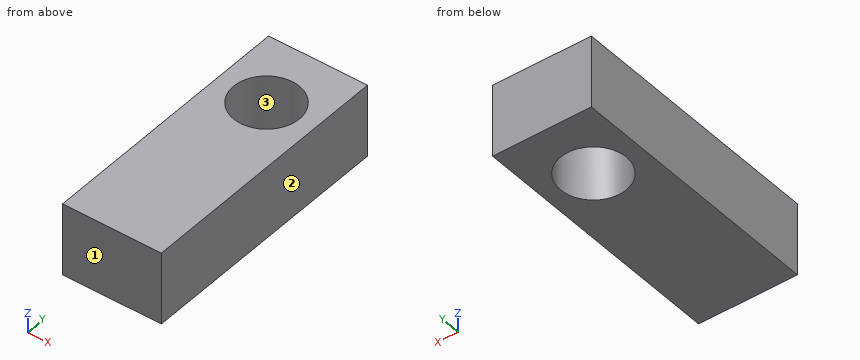
Autodesk Inventor part; units mm, degrees
ref_plane "YZ Plane" through (0, 0, 0) normal (1, 0, 0) x (0, 1, 0)
ref_plane "XZ Plane" through (0, 0, 0) normal (0, 1, 0) x (-1, 0, 0)
ref_plane "XY Plane" through (0, 0, 0) normal (0, 0, 1) x (1, 0, 0)
sketch "Sketch1" plane through (0, 0, 0) normal (0, 0, 1) x (1, 0, 0)
  line L0 (-7.5, 40) -> (7.5, 40)
  line L1 (7.5, 40) -> (7.5, 0)
  line L2 (7.5, 0) -> (-7.5, 0)
  line L3 (-7.5, 0) -> (-7.5, 40)
  line L4 (-10.7602, 0) -> (12.0613, 0)
  line L5 (0, -8) -> (0, 48)
  point P0 (0, 0)
  dimension "d4" = 7.5
  dimension "d5" = 7.5
  dimension "d6" = 40
  dimension "d7" = 0
extrude "Extrusion1" add sketch "Sketch1" along normal blind 11
sketch "Sketch3" plane through (-7.5, 0, 0) normal (0, -1, 0) x (1, 0, 0)
  line L0 (0, 0) -> (0, 11)
  line L1 (0, 5.5) -> (13.8011, 5.5)
  line L2 (0, 11) -> (15, 11)
  circle A0 centre (5, 5.5) radius 1
  point P0 (7.5, 0)
  dimension "d11" = 5.5
  dimension "d12" = 2
sketch "Sketch4" plane through (0, 0, 11) normal (0, 0, 1) x (1, 0, 0)
  circle A0 centre (0, 30) radius 5
  line L0 (-7.5, 0) -> (7.5, 0)
  point P0 (0, 0)
  dimension "d13" = 10
  dimension "d14" = 30
extrude "Extrusion3" cut sketch "Sketch4" against normal through all
properties part number "mallet_support"
The model under review builds one solid part; all positions refer to its coordinate system, in mm. Face numbers are marked on the shaded views. Round coordinates to 2 decimals unless told otherwise and drop trailing zeros. Loops run counter-clockwise (first coordinate to the right, second up) from the corner with the lowest first, then second, coordinate; pieces in that order, holes last. Notation, with made-up numbers: (43, 1) -> (94, 1) arc R21 cw to (94, 17) -> close; hole circle Ø1 at (-4, -24). An arc over 180 degrees is marked (long way). Answer as CSV lines item,"result".
1) To check wall thickness, follow line 1 along Y through (x, z) = (0.25, 5.5); line 2 along Y through (x, z) = (-3.5, 1.25); line 3 along X through (y, z) = (29.5, 7.25). State the ranges of each line that lie inside material, in increasing order. Write a range as from..to.
Geometry results:
line 1,"y = 0..25.01, 34.99..40"
line 2,"y = 0..26.43, 33.57..40"
line 3,"x = -7.5..-4.97, 4.97..7.5"
2) Add section A-A on z = 1.5. Write out the cut boundary in (x, y).
Geometry results:
outline,"(-7.5, 0) -> (7.5, 0) -> (7.5, 40) -> (-7.5, 40) -> close; hole circle Ø10 at (0, 30)"
3) Add section B-B on y = 30. Write out the cut boundary in (x, z).
Geometry results:
outline,"(-7.5, 0) -> (-5, 0) -> (-5, 11) -> (-7.5, 11) -> close; (5, 0) -> (7.5, 0) -> (7.5, 11) -> (5, 11) -> close"
4) Add section C-C on x = 0. Write out the cut boundary in (y, z).
Geometry results:
outline,"(0, 0) -> (25, 0) -> (25, 11) -> (0, 11) -> close; (35, 0) -> (40, 0) -> (40, 11) -> (35, 11) -> close"
5) Draft analysis for pull direction Y (two halves, no side actions). For the marked faces 1, 2 and 3, state which applies: pulls with the +Y half, pulls with the -Y half, needs draft (parallel to the pull), parting line crosses it, or undercut.
Geometry results:
face 1,"pulls with the -Y half"
face 2,"needs draft"
face 3,"undercut"
